Part model, mm, in its own coordinate system. A direction names the side the tool comes from. Coordinates: 2 decimals unless noted, no trailing zeros. Order: outer loops, then holes, each group sorted by start corner. A loop starts at its lowest first (then second) coordinate and runs counter-clockwise, first axis right, second up.
```python
from build123d import *

# Parameters (mm, degrees)
F0_R     = 1.5
F1_DEPTH = 15
F2_DEPTH = 20
F3_SIZE  = 0.2
F4_DEPTH = 2.5


# Not quite as in the source:
# - a feature names something its author has since deleted; it is built from what else it names


with BuildPart() as f1:
    # F0 (on Top) → F1 (new body)
    with BuildSketch(Plane.XY):
        Polygon((-6.5392298422, -1.443375673), (-6.5392298422, 1.443375673), (-9.0392298422, 2.8867513459), (-11.5392298422, 1.443375673), (-11.5392298422, -1.443375673), (-9.0392298422, -2.8867513459), align=None)
        with Locations((-9.0392298422, 0)):
            Circle(F0_R, mode=Mode.SUBTRACT)
    extrude(amount=F1_DEPTH)

    # F0 (on Top) → F2 (join)
    with BuildSketch(Plane.XY):
        with Locations((-9.0392298422, 0)):
            Circle(F0_R)
    extrude(amount=F2_DEPTH)

    # F3
    f3_edges = [f1.edges().sort_by_distance(p)[0] for p in [
        (-10.53923, 0, 20),
    ]]
    chamfer(f3_edges, length=F3_SIZE)

    # F0 (on Top) → F4 (cut)
    with BuildSketch(Plane.XY):
        with Locations((-9.0392298422, 0)):
            Circle(F0_R)
    extrude(amount=F4_DEPTH, mode=Mode.SUBTRACT)


solid = f1.part
```
(1) Slice it at A-A, the plane y = 0. Give the cut face in (x, z).
(2) Slice it at C-C, the plane z = 6. Give the cut face in (x, y), then the cut area to 3 significant figures.
(3) Slice it at D-D, the plane x = -7.1. Give the cut face in (y, z), then the cut area to 3 significant figures.
(4) Pull direction X, two halves, no side cores. Call faces 3 (the face through (-7.772, 2.155, 7.395)), 4 (the face through (-10.2, -1.2, 15)), 5 (the face through (-10.538, 0.066, 17.366)), 6 (the face through (-10.538, 0.066, 1.232)): +X half, -X half, draft (parallel to the pull), parting line (faces both ways), or undercut.
(5) Slice it at B-B, the plane z = 15.5. Give the cut face in (x, y).
(6) Probe line 1 (Z direction, x = -7.1, y = 0.4); line 2 (Y direction, x = -10.25, z = 2); line 3 (Z direction, x = -8.35, y = 0.6). List the from-to ranges inside material, lowest first.
(7) Tool access for faces 1 (the face through (-9, 0, 2.5)), 2 (the face through (-7.807, -2.175, 7.395)): list every direction of +Z, -Z, +X, -X, +Y, -Y with a clear straight run to the whole face (end or side of a thin tool).
(8) Drop a flat-ended pin along its axis: pin 1 (1 mm diameter, centred on y = 1.5, z = 17, fed in from -X). Give the stop position or say it passes through.
Here are the results:
1. outline: (-11.54, 0) - (-10.54, 0) - (-10.54, 2.5) - (-7.54, 2.5) - (-7.54, 0) - (-6.54, 0) - (-6.54, 15) - (-7.54, 15) - (-7.54, 19.8) - (-7.74, 20) - (-10.34, 20) - (-10.54, 19.8) - (-10.54, 15) - (-11.54, 15) - close
2. outline: (-11.54, -1.44) - (-9.04, -2.89) - (-6.54, -1.44) - (-6.54, 1.44) - (-9.04, 2.89) - (-11.54, 1.44) - close
2. area: 21.7 mm2
3. outline: (-1.77, 0) - (1.77, 0) - (1.77, 15) - (-1.77, 15) - close
3. area: 53.0 mm2
4. face 3: +X half
4. face 4: draft
4. face 5: parting line
4. face 6: undercut
5. outline: circle Ø3 at (-9.04, 0)
6. line 1: z = 0 to 15
6. line 2: y = -2.19 to -0.89, 0.89 to 2.19
6. line 3: z = 2.5 to 20
7. face 1: -Z
7. face 2: +Z, -Z, +X, -Y
8. pin 1: stops at x = -10.16
